Design review of the part built by this model. Coordinates are the model's own, in mm. Face numbers are marked on the shaded views. A direction names the side the tool comes from. Give positions to 0.01 mm unless a question says otherwise; leave off trailing zeros. Order: outer loops, then holes, each group sorted by start corner. A loop starts at its lowest first (then second) coordinate and runs counter-clockwise, first axis right, second up. Notation, with made-up numbers: (61, 9) -> (71, 9) arc R22 ccw to (71, 29) -> close; hole circle Ø6 at (65, 2.25). An arc over 180 degrees is marked (long way). One line per item, written item: value. Start each with the question number.
1) Consider section C-C (x = -32.5). State the section outline as (y, z) points.
2) Consider section D-D (x = 31.5). State the section outline as (y, z) points, plus the area to 3 significant figures.
3) For pin 1 (5 mm diameter, centred on x = -4.5, y = -58.5, fed in from -Z); pin 2 (6.5 mm diameter, centred on x = 55, y = -34, fed in from +Z); pin 3 (1.5 mm diameter, centred on x = -32.5, z = 9, fed in from -Y), all flat-tipped, find the tip position at first contact; note any pin that passes through.
4) Consider section A-A (z = 12.5). State the section outline as (x, y) points.
5) Wall thickness on line 1 along X through (y, z) = (-56, 18.75); line 2 along X through (y, z) = (-6, 5); line 3 along Y through (x, z) = (43, 19): over which ranges is each line inside the solid? List them lowest first. Write a range as from..to.
6) Tool access review of the marked faces 1, 2 and 3: name each direction out of +Z, -Z, +X, -X, +Y, -Y from which nothing blocks a thin tool from reaching the whole face with its end or side.
7) Consider section B-B (y = -48.5). State the section outline as (x, z) points.
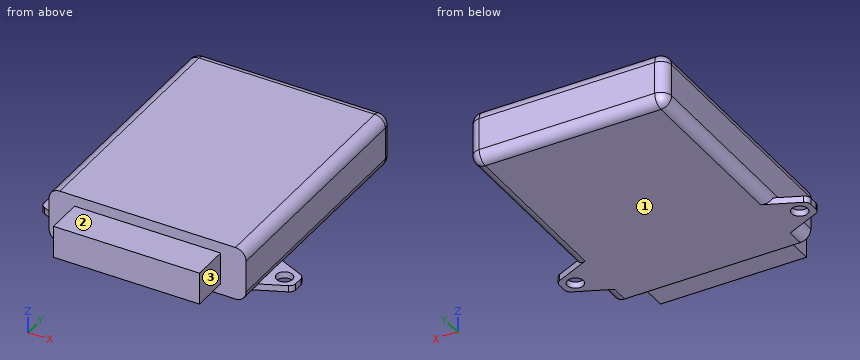
from build123d import *

# Parameters (mm, degrees)
EXTRUDE_1_DEPTH = 25
FILLET_2_R      = 5
FILLET_3_R      = 5
SKETCH_2_W      = 68.2
SKETCH_2_H      = 15
EXTRUDE_2_DEPTH = 17
SKETCH_3_R      = 3.75
EXTRUDE_3_DEPTH = 3


with BuildPart() as part:
    # 草图1 → 凸台-拉伸1 (new body)
    with BuildSketch(Plane.XY):
        with BuildLine():
            Line((-37.933333333, 65.994666667), (44.066666667, 65.994666667))
            ThreePointArc((44.066666667, 65.994666667), (47.602200573, 64.530200573), (49.066666667, 60.994666667))
            Line((49.066666667, 60.994666667), (49.066666667, -51.305333333))
            Line((49.066666667, -51.305333333), (-42.933333333, -51.305333333))
            Line((-42.933333333, -51.305333333), (-42.933333333, 60.994666667))
            ThreePointArc((-42.933333333, 60.994666667), (-41.468867239, 64.530200573), (-37.933333333, 65.994666667))
        make_face()
    extrude(amount=EXTRUDE_1_DEPTH)

    # 圆角2
    fillet_2_edges = [part.edges().sort_by_distance(p)[0] for p in [
        (47.602200573, 64.530200573, 25),
        (49.066666667, 4.844666667, 25),
        (-42.933333333, 4.844666667, 25),
        (-41.468867239, 64.530200573, 25),
        (3.066666667, 65.994666667, 25),
    ]]
    fillet(fillet_2_edges, radius=FILLET_2_R)

    # 圆角3
    fillet_3_edges = [part.edges().sort_by_distance(p)[0] for p in [
        (-42.933333333, 4.844666667, 0),
        (49.066666667, 4.844666667, 0),
        (47.602200573, 64.530200573, 0),
        (3.066666667, 65.994666667, 0),
        (-41.468867239, 64.530200573, 0),
    ]]
    fillet(fillet_3_edges, radius=FILLET_3_R)

    # 草图2 → 凸台-拉伸2 (add)
    with BuildSketch(Plane.XZ.offset(51.305333333)):
        with Locations((3.066666667, 12.5)):
            Rectangle(SKETCH_2_W, SKETCH_2_H)
    extrude(amount=EXTRUDE_2_DEPTH)

    # 草图3 → 凸台-拉伸3 (add)
    with BuildSketch(Plane(origin=(0, 0, 0), x_dir=(-1, 0, 0), z_dir=(0, 0, -1))):
        with BuildLine():
            Line((-60.065426781, -26.521117388), (-43.846003667, -19.305333333))
            Line((-43.846003667, -19.305333333), (-43.846003667, -31.305333333))
            Line((-43.846003667, -31.305333333), (-43.846003667, -43.305333333))
            Line((-43.846003667, -43.305333333), (-60.063408173, -36.104747529))
            ThreePointArc((-60.063408173, -36.104747529), (-61.361177964, -34.998068142), (-61.846002246, -33.362864452))
            Line((-61.846002246, -33.362864452), (-61.846002246, -29.262103306))
            ThreePointArc((-61.846002246, -29.262103306), (-61.36177982, -27.62782573), (-60.065426781, -26.521117388))
        make_face()
        with Locations((-55.456334457, -31.312483879)):
            Circle(SKETCH_3_R, mode=Mode.SUBTRACT)
    extrude_3 = extrude(amount=-EXTRUDE_3_DEPTH)

    # 镜向1: 凸台-拉伸3 across plane
    add(extrude_3.mirror(Plane(origin=(3.066666667, 0, 0), x_dir=(0, 0, 1), z_dir=(1, 0, 0))))


solid = part.part
Checked values:
1. outline: (-51.31, 0) -> (60.99, 0) arc R5 ccw to (65.99, 5) -> (65.99, 20) arc R5 ccw to (60.99, 25) -> (-51.31, 25) -> close
2. outline: (-68.31, 5) -> (-51.31, 5) -> (-51.31, 0) -> (60.99, 0) arc R5 ccw to (65.99, 5) -> (65.99, 20) arc R5 ccw to (60.99, 25) -> (-51.31, 25) -> (-51.31, 20) -> (-68.31, 20) -> close
2. area: 3,180 mm^2
3. pin 1: stops at z = 5
3. pin 2: stops at z = 3
3. pin 3: stops at y = -51.31
4. outline: (-42.93, -51.31) -> (-31.03, -51.31) -> (-31.03, -68.31) -> (37.17, -68.31) -> (37.17, -51.31) -> (49.07, -51.31) -> (49.07, 60.99) arc R5 ccw to (44.07, 65.99) -> (-37.93, 65.99) arc R5 ccw to (-42.93, 60.99) -> close
5. line 1: x = -31.03..37.17
5. line 2: x = -42.93..49.07
5. line 3: y = -51.31..65.99
6. face 1: -Z, +X, -X, +Y, -Y
6. face 2: +Z, +X, -X, -Y
6. face 3: +Z, -Z, +X, -Y
7. outline: (-42.93, 5) arc R5 ccw to (-37.93, 0) -> (44.07, 0) arc R5 ccw to (49.07, 5) -> (49.07, 20) arc R5 ccw to (44.07, 25) -> (-37.93, 25) arc R5 ccw to (-42.93, 20) -> close
